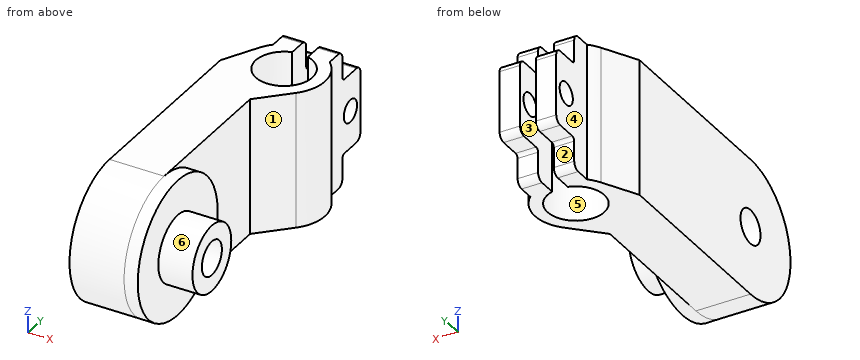
```python
from build123d import *

# Parameters (mm, degrees)
EXTRUDE_1_DEPTH             = 10
SKETCH_6_R                  = 1.65
SKETCH_6_W                  = 14.704506527
SKETCH_6_H                  = 8.520368268
CUT_EXTRUDE_2_DEPTH         = 34.876577454
FILLET_1_R                  = 1
FILLET_2_R                  = 0.5
EXTRUDE_2_REACH             = 34.619
SKETCH_7_R                  = 10
EXTRUDE_2_DIRECTION_2_DEPTH = 2
SKETCH_8_R                  = 4.85
EXTRUDE_3_DEPTH             = 5
SKETCH_9_R                  = 2.5
CUT_EXTRUDE_3_DEPTH         = 44.874821937


with BuildPart() as part:
    # 草图1 → 凸台-拉伸1 (new, symmetric)
    with BuildSketch(Plane.XY):
        with BuildLine():
            Line((-1.15, 3.987480407), (-1.15, 12))
            Line((-1.15, 12), (-4.15, 12))
            Line((-4.15, 12), (-4.15, 4.333301282))
            ThreePointArc((-4.15, 4.333301282), (-4.784308974, 3.620826928), (-5.297685557, 2.816829377))
            Line((-5.297685557, 2.816829377), (-8, -2.265484914))
            Line((-8, -2.265484914), (-8, -30))
            Line((-8, -30), (0, -30))
            Line((0, -30), (0, -8.485281374))
            Line((0, -8.485281374), (4.242640687, -4.242640687))
            ThreePointArc((4.242640687, -4.242640687), (5.999649956, 0.064810571), (4.15, 4.333301282))
            Line((4.15, 4.333301282), (4.15, 12))
            Line((4.15, 12), (1.15, 12))
            Line((1.15, 12), (1.15, 3.987480407))
            ThreePointArc((1.15, 3.987480407), (0, -4.15), (-1.15, 3.987480407))
        make_face()
    extrude(amount=EXTRUDE_1_DEPTH, both=True)

    # 草图6 → 切除-拉伸2 (cut, through all)
    with BuildSketch(Plane(origin=(4.15, 0, 0), x_dir=(0, 0, -1), z_dir=(1, 0, 0))):
        with Locations(Location((0, 9.5, 0), (0, 0, 90))):
            Circle(SKETCH_6_R)
        with Locations((-12.852253263, 11.760184134)):
            Rectangle(SKETCH_6_W, SKETCH_6_H)
        with Locations((12.852253263, 11.760184134)):
            Rectangle(SKETCH_6_W, SKETCH_6_H)
    extrude(amount=-CUT_EXTRUDE_2_DEPTH, mode=Mode.SUBTRACT)

    # 圆角1
    fillet_1_edges = [part.edges().sort_by_distance(p)[0] for p in [
        (2.65, 7.5, -10),
        (-2.65, 7.5, -10),
        (2.65, 7.5, 10),
        (-2.65, 7.5, 10),
        (2.65, 12, 5.5),
        (-2.65, 12, 5.5),
        (2.65, 12, -5.5),
        (-2.65, 12, -5.5),
    ]]
    fillet(fillet_1_edges, radius=FILLET_1_R)

    # 圆角2
    fillet_2_edges = [part.edges().sort_by_distance(p)[0] for p in [
        (-2.65, 7.5, 5.5),
        (2.65, 7.5, 5.5),
        (2.65, 7.5, -5.5),
        (-2.65, 7.5, -5.5),
    ]]
    fillet(fillet_2_edges, radius=FILLET_2_R)

    # 凸台-拉伸2: up to this face of the body (flat: up to its plane)
    extrude_2_end = Plane(part.part.faces().sort_by_distance((-8, -16.132742457, 0))[0])
    # 草图7 → 凸台-拉伸2 (add, up to the picked face)
    with BuildSketch(Plane(origin=(0, 0, 0), x_dir=(0, 0, -1), z_dir=(1, 0, 0)), mode=Mode.PRIVATE) as extrude_2_sk1:
        with Locations(Location((0, -30, 0), (0, 0, 180))):
            Circle(SKETCH_7_R)
    extrude_2_tool1 = split(extrude(extrude_2_sk1.sketch, amount=-EXTRUDE_2_REACH, mode=Mode.PRIVATE), bisect_by=extrude_2_end, keep=Keep.BOTH, mode=Mode.PRIVATE)
    add(extrude_2_tool1.solids().sort_by(Axis((0, -30, 0), (-1, 0, 0)))[0])

    # 草图7 → 凸台-拉伸2 direction 2 (add)
    with BuildSketch(Plane(origin=(0, 0, 0), x_dir=(0, 0, -1), z_dir=(1, 0, 0))):
        with Locations(Location((0, -30, 0), (0, 0, 180))):
            Circle(SKETCH_7_R)
    extrude(amount=EXTRUDE_2_DIRECTION_2_DEPTH)

    # 草图8 → 凸台-拉伸3 (add)
    with BuildSketch(Plane(origin=(2, 0, 0), x_dir=(0, 0, -1), z_dir=(1, 0, 0))):
        with Locations(Location((0, -30, 0), (0, 0, 90))):
            Circle(SKETCH_8_R)
    extrude(amount=EXTRUDE_3_DEPTH)

    # 草图9 → 切除-拉伸3 (cut, through all)
    with BuildSketch(Plane(origin=(7, 0, 0), x_dir=(0, 0, -1), z_dir=(1, 0, 0))):
        with Locations(Location((0, -30, 0), (0, 0, 90))):
            Circle(SKETCH_9_R)
    extrude(amount=-CUT_EXTRUDE_3_DEPTH, mode=Mode.SUBTRACT)


solid = part.part
```
Can you work these out from the model? Positions are in its coordinate system, mm. Face numbers are marked on the shaded views. A direction names the side the tool comes from. Give positions to 0.01 mm unless a question says otherwise; leave off trailing zeros. Loops run counter-clockwise (first coordinate to the right, second up) from the corner with the lowest first, then second, coordinate; pieces in that order, holes last. Notation, with made-up numbers: M 35,30.25 L 85,30.25 A29 cw 85,50.25 Z; hole C -29,51 d5. An arc over 180 degrees is marked long. Answer in a Markdown table with one row per item.
1. Suppose I cut it at A-A on x = 3.5. Write out the boundary of the cut face in (y, z).
Taken from the geometry:
| item | result |
|---|---|
| outline | C -30,0 d9.7; M -4.99,-10 L -2.23,-10 L -2.23,10 L -4.99,10 Z; M 2.23,-10 L 6.5,-10 A1 ccw 7.5,-9 L 7.5,-6 A0.5 cw 8,-5.5 L 11,-5.5 A1 ccw 12,-4.5 L 12,4.5 A1 ccw 11,5.5 L 8,5.5 A0.5 cw 7.5,6 L 7.5,9 A1 ccw 6.5,10 L 2.23,10 Z; hole C -30,0 d5; hole C 9.5,0 d3.3 |
2. Suppose I cut it at C-C on z = -3.25. Write out the boundary of the cut face in (x, y), plus the area to 3 significant figures.
Taken from the geometry:
| item | result |
|---|---|
| outline | M -8,-39.46 L 2,-39.46 L 2,-33.6 L 7,-33.6 L 7,-26.4 L 2,-26.4 L 2,-20.54 L 0,-20.54 L 0,-8.49 L 4.24,-4.24 A6 ccw 4.15,4.33 L 4.15,12 L 1.15,12 L 1.15,3.99 A4.15 cw long -1.15,3.99 L -1.15,12 L -4.15,12 L -4.15,4.33 A6 ccw -5.3,2.82 L -8,-2.27 Z |
| area | 459 mm² |
3. If I drill on line 1 along Z through (x, y) = (-3.75, -30); line 2 along Z through (x, y) = (-1.85, 9.5); line 3 along Y through (x, z) = (-2, 1.5), over which ranges is the centre line in solid material (lowest first)?
Taken from the geometry:
| item | result |
|---|---|
| line 1 | z = -10 to -2.5, 2.5 to 10 |
| line 2 | z = -5.5 to -1.65, 1.65 to 5.5 |
| line 3 | y = -39.89 to -32, -28 to -3.64, 3.64 to 8.81, 10.19 to 12 |
4. Which directions (+Z, -Z, +X, -X, +Y, -Y) give clear straight access to the entire face, cutting with the end or side of a thin tool? Please do the marked faces 1, 2 and 3.
Taken from the geometry:
| item | result |
|---|---|
| face 1 | +Z, -Z, +X |
| face 2 | -Z, +X, -X, +Y |
| face 3 | +Z, -Z, +Y |
5. For pin 1 Ø4 at (y, z) = (9, 3) entering from +X; pin 2 Ø1 at (y, z) = (-13, -2.5) entering from +X; pin 3 Ø1.5 at (x, z) = (-2.5, -7) entering from +Y, each with a flat end and sliding along its axis, tell me the tip position at first contact or that it passes through.
Taken from the geometry:
| item | result |
|---|---|
| pin 1 | stops at x = 4.15 |
| pin 2 | stops at x = 0 |
| pin 3 | stops at y = 7.5 |
6. Suppose I cut it at B-B on y = 9.5. Write out the boundary of the cut face in (x, z), plus the area to 3 significant figures.
Taken from the geometry:
| item | result |
|---|---|
| outline | M -4.15,-5.5 L -1.15,-5.5 L -1.15,-1.65 L -4.15,-1.65 Z; M -4.15,1.65 L -1.15,1.65 L -1.15,5.5 L -4.15,5.5 Z; M 1.15,-5.5 L 4.15,-5.5 L 4.15,-1.65 L 1.15,-1.65 Z; M 1.15,1.65 L 4.15,1.65 L 4.15,5.5 L 1.15,5.5 Z |
| area | 46.2 mm² |
7. Suppose I cut it at D-D on x = -6.75. Write out the boundary of the cut face in (y, z).
Taken from the geometry:
| item | result |
|---|---|
| outline | M -30,-10 L 0.09,-10 L 0.09,10 L -30,10 A10 ccw Z; hole C -30,0 d5 |
8. Thinking about a two-plate mould opening in X: for the marked faces 4, 5 and 6, which applies, released by +X, released by -X, zero draft, split by the parting line, or undercut?
Taken from the geometry:
| item | result |
|---|---|
| face 4 | released by -X |
| face 5 | undercut |
| face 6 | zero draft |
